Verification items for the finished model (mm, model axes). Face numbers are marked on the shaded views. A direction names the side the tool comes from. Coordinates: 2 decimals unless noted, no trailing zeros. Loops run counter-clockwise (first coordinate to the right, second up) from the corner with the lowest first, then second, coordinate; pieces in that order, holes last. Notation, with made-up numbers: (38.5, 70) -> (62.5, 70) arc R16 cw to (62.5, 75) -> close; hole circle Ø11 at (-21, 27.25). An arc over 180 degrees is marked (long way). Answer as a JSON object with one key per item and string values. Group by question number.
Q1. Cross-section at B-B on y = 11. Record the boundary of the cut face in (x, z), and give its area (3 significant figures).
Q2. Cross-section at C-C on y = 2. Record the boundary of the cut face in (x, z), and give its area (3 significant figures).
Q3. Scan lines: L1, parallel to Y at x = 0, z = 5.75; L2, parallel to Z at x = -7, y = 1.5; L3, parallel to Z at x = 13.5, y = 6. Record each from-to range of solid material in increasing order.
Q4. Set-up check for the marked faces 1 and 2: record each of +Z, -Z, +X, -X, +Y, -Y from which the full face is reachable in a straight line by a thin tool's end or side.
Q5. Cross-section at A-A on x = 11. Record the boundary of the cut face in (y, z).
Q6. Release check for a two-part mould opening along X. For the marked faces 3, 4 and 5 record: released by +X, released by -X, zero draft, split by the parting line, or undercut.
Q7. Gauge pin test, flat ends, axial feed: pin 1 Ø8 at (y, z) = (2, 23) entering from -X; pin 2 Ø3 at (x, y) = (0, 0) entering from +Z; pin 3 Ø1 at (y, z) = (8, 34) entering from -X. Record the tip position at first contact, or that the pin passes through.
```python
from build123d import *

# Parameters (mm, degrees)
F0_W        = 30
F0_H        = 30
F1_DEPTH    = 7
F2_W        = 10
F2_H        = 30
F3_DEPTH    = 35
F4_T1_DEPTH = 81.4336597593
F5_W        = 25.2
F5_H        = 25.2
F6_DEPTH    = 2
F9_D        = 2.5
F9_DEPTH    = 16.5
F9_TIP      = 0.7510757738
F10_W       = 20.2
F10_H       = 6.5
F11_DEPTH   = 1
F14_D       = 1.5
F16_D       = 3


# Not quite as in the source:
# - a fillet or chamfer that OpenCascade refuses, or shapes differently, is made with other operations: its cross-section is extruded or revolved along the edge and cut away or added


with BuildPart() as f1:
    # F0 (on Top) → F1 (new body)
    with BuildSketch(Plane.XY):
        Rectangle(F0_W, F0_H)
    extrude(amount=F1_DEPTH)

    # F2 (on face) → F3 (join)
    with BuildSketch(Plane.XY.offset(7)):
        Rectangle(F2_W, F2_H)
    extrude(amount=F3_DEPTH)

    # F4: chamfer of 10 on 1 edges, made by hand

    # F4_s2 → F4_t1 (cut)
    with BuildSketch(Plane.XZ.offset(-40.7168298797)):
        Polygon((-5, 32), (5, 42), (-5, 42), align=None)
    extrude(amount=F4_T1_DEPTH, mode=Mode.SUBTRACT)


with BuildPart() as f6:
    # F5 (on face) → F6 (new body)
    with BuildSketch(Plane(origin=(0, 0, 0), x_dir=(1, 0, 0), z_dir=(0, 0, -1))):
        Rectangle(F5_W, F5_H)
    extrude(amount=-F6_DEPTH)


with BuildPart() as f1_1:
    add(f1.part)

    # F7: cut F6
    add(f6.part, mode=Mode.SUBTRACT)

    # F9
    with Locations(Plane(origin=(0, 0, 2), x_dir=(1, 0, 0), z_dir=(0, 0, -1))):
        with Locations((0, 0)):
            Hole(F9_D / 2, depth=F9_DEPTH)
            with Locations((0, 0, -(F9_DEPTH + F9_TIP / 2))):  # 118° drill point
                Cone(0, F9_D / 2, F9_TIP, mode=Mode.SUBTRACT)


with BuildPart() as f11:
    # F10 (on face) → F11 (new body)
    with BuildSketch(Plane(origin=(-18.5, 0, 18.5), x_dir=(0, -1, 0), z_dir=(-0.7071067812, 0, 0.7071067812))):
        with Locations((0, 29.9840187158)):
            Rectangle(F10_W, F10_H)
    extrude(amount=-F11_DEPTH)


with BuildPart() as f1_2:
    add(f1_1.part)

    # F12: cut F11
    add(f11.part, mode=Mode.SUBTRACT)

    # F14 (through all)
    with Locations(Plane(origin=(-17.7928932188, 0, 17.7928932188), x_dir=(0, -1, 0), z_dir=(-0.7071067812, 0, 0.7071067812))):
        with Locations((-8, 30.2340187158), (8, 30.2340187158)):
            Hole(F14_D / 2)

    # F16 (through all)
    with Locations(Plane(origin=(-18.5, 0, 18.5), x_dir=(0, -1, 0), z_dir=(-0.7071067812, 0, 0.7071067812))):
        with Locations((-10, 22.091883092), (10, 22.091883092)):
            Hole(F16_D / 2)


solid = f1_2.part
```
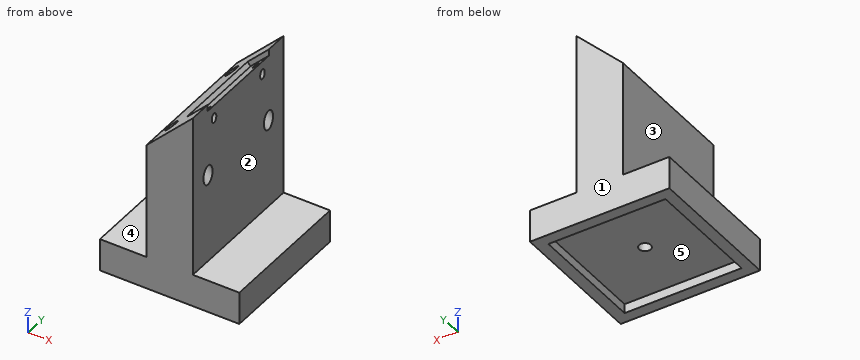
Computed values:
{
 "1": {"outline": "(-15, 0) -> (-12.6, 0) -> (-12.6, 2) -> (12.6, 2) -> (12.6, 0) -> (15, 0) -> (15, 7) -> (5, 7) -> (5, 24.66) -> (-3.67, 33.33) -> (-5, 32) -> (-5, 7) -> (-15, 7) -> close; (-2.09, 34.91) -> (5, 27.82) -> (5, 42) -> close", "area": "435 mm²"},
 "2": {"outline": "(-15, 0) -> (-12.6, 0) -> (-12.6, 2) -> (12.6, 2) -> (12.6, 0) -> (15, 0) -> (15, 7) -> (5, 7) -> (5, 40.59) -> (1.11, 36.7) -> (0.4, 37.4) -> (-5, 32) -> (-5, 7) -> (-15, 7) -> close", "area": "454 mm²"},
 "3": {"L1": "y = -15 to -1.25, 1.25 to 15", "L2": "z = 2 to 7", "L3": "z = 0 to 7"},
 "4": {"face 1": "+Z, -Z, +X, -X, +Y", "face 2": "+Z, +X, +Y, -Y"},
 "5": {"outline": "(-15, 0) -> (-12.6, 0) -> (-12.6, 2) -> (12.6, 2) -> (12.6, 0) -> (15, 0) -> (15, 7) -> (-15, 7) -> close"},
 "6": {"face 3": "released by -X", "face 4": "zero draft", "face 5": "undercut"},
 "7": {"pin 1": "stops at x = -5", "pin 2": "stops at z = 37.4", "pin 3": "stops at x = -3.5"}
}
